Read the model definition and answer for the solid it produces. Units are mm, in the model's axes. A direction names the side the tool comes from. Round coordinates to 2 decimals unless told otherwise and drop trailing zeros. Write each loop counter-clockwise with the first axis right and the second up, starting at its lowest first coordinate (ties: lowest second). Pieces come first, ordered by that corner, then holes. Notation, with made-up numbers: (34, 14.25) - (54, 14.25) arc R25 cw to (54, 35.25) - close; hole circle Ø1 at (-36.75, 25.5). An arc over 180 degrees is marked (long way). One line per item, written item: value. Start each with the question number.
(1) A cutting plane is placed at A-A, the plane x = 9.5. State how many separate pieces and enclosed holes the cut face has, plus the area to 3 significant figures.
(2) Find the intervals of material crossed by L1, parallel to Y at x = 80, z = 93.5; L2, parallel to X at y = 147, z = 83; L3, parallel to Z at x = 20, y = 40.5, in increasing order.
(3) The mould has two halves that part along Y. Classify faces 3 (the face through (76, 85, 33)), 4 (the face through (0, 78, 63)), 5 (the face through (41, 0, 63)): +Y half, -Y half, draft (parallel to the pull), parting line (faces both ways), or undercut.
(4) A cutting plane is placed at D-D, the plane x = 68. Determine the outline of the cut face in (y, z).
(5) A cutting plane is placed at C-C, the plane y = 125.5. Determine the outline of the cut face in (x, z), plus the area to 3 significant figures.
(6) A cutting plane is placed at B-B, the plane z = 8. Determine the outline of the cut face in (x, y), plus the area to 3 significant figures.
(7) For faces 1 (the face through (76, 124, 33)), 2 (the face through (41, 157.8, 63)), determine the directions among +Z, -Z, +X, -X, +Y, -Y from which every point of the face is accessible in a straight line to the end or side of a thin tool.
(8) Flat-ended cylindrical pins translate along their axes: pin 1 Ø11 at (x, y) = (74, 125.5) entering from +Z; pin 2 Ø12 at (x, y) = (43, 129) entering from +Z; pin 3 Ø1.5 at (x, y) = (44, 1) entering from +Z. Find the tip coordinate at first contact, or state that the pin passes through.
from build123d import *

# Parameters (mm, degrees)
SKETCH1_W           = 83.5
SKETCH1_H           = 157.8
SKETCH1_W_2         = 77.5
SKETCH1_H_2         = 35.7
BOSS_EXTRUDE1_DEPTH = 123
SKETCH1_3_W         = 77.5
SKETCH1_3_H         = 35.7
BOSS_EXTRUDE2_DEPTH = 3
SKETCH2_W           = 77.5
SKETCH2_H           = 27
CUT_EXTRUDE1_DEPTH  = 100
SKETCH4_W           = 3
SKETCH4_H           = 10
BOSS_EXTRUDE3_DEPTH = 10
SKETCH5_W           = 3
SKETCH5_H           = 10
BOSS_EXTRUDE4_DEPTH = 10
SKETCH7_W           = 3
SKETCH7_H           = 157.8
BOSS_EXTRUDE5_DEPTH = 5
SKETCH8_W           = 1
SKETCH8_H           = 2.5
CUT_EXTRUDE2_DEPTH  = 154.8
SKETCH9_W           = 7.5
SKETCH9_H           = 7.5
CUT_EXTRUDE3_DEPTH  = 10


with BuildPart() as part:
    # Sketch1 → Boss-Extrude1 (new body)
    with BuildSketch(Plane.XY):
        with Locations((41.75, 78.9)):
            Rectangle(SKETCH1_W, SKETCH1_H)
        with Locations((41.75, 20.85)):
            Rectangle(SKETCH1_W_2, SKETCH1_H_2, mode=Mode.SUBTRACT)
        with Locations((41.75, 59.55)):
            Rectangle(SKETCH1_W_2, SKETCH1_H_2, mode=Mode.SUBTRACT)
        with Locations((41.75, 98.25)):
            Rectangle(SKETCH1_W_2, SKETCH1_H_2, mode=Mode.SUBTRACT)
        with Locations((41.75, 136.95)):
            Rectangle(SKETCH1_W_2, SKETCH1_H_2, mode=Mode.SUBTRACT)
    extrude(amount=BOSS_EXTRUDE1_DEPTH)

    # Sketch1<3> → Boss-Extrude2 (add)
    with BuildSketch(Plane.XY):
        with Locations((41.75, 136.95)):
            Rectangle(SKETCH1_3_W, SKETCH1_3_H)
        with Locations((41.75, 98.25)):
            Rectangle(SKETCH1_3_W, SKETCH1_3_H)
        with Locations((41.75, 59.55)):
            Rectangle(SKETCH1_3_W, SKETCH1_3_H)
        with Locations((41.75, 20.85)):
            Rectangle(SKETCH1_3_W, SKETCH1_3_H)
    extrude(amount=BOSS_EXTRUDE2_DEPTH)

    # Sketch2 → Cut-Extrude1 (cut)
    with BuildSketch(Plane(origin=(0, 119.1, 0), x_dir=(1, 0, 0), z_dir=(0, 1, 0))):
        with Locations((41.75, -16.5)):
            Rectangle(SKETCH2_W, SKETCH2_H)
    extrude(amount=-CUT_EXTRUDE1_DEPTH, mode=Mode.SUBTRACT)

    # Sketch4 → Boss-Extrude3 (add)
    with BuildSketch(Plane(origin=(3, 0, 0), x_dir=(0, 0, -1), z_dir=(1, 0, 0))):
        with Locations((-31.5, 85.4)):
            Rectangle(SKETCH4_W, SKETCH4_H)
        with Locations((-31.5, 124.1)):
            Rectangle(SKETCH4_W, SKETCH4_H)
        with Locations((-31.5, 46.7)):
            Rectangle(SKETCH4_W, SKETCH4_H)
        with Locations((-31.5, 8)):
            Rectangle(SKETCH4_W, SKETCH4_H)
    extrude(amount=BOSS_EXTRUDE3_DEPTH)

    # Sketch5 → Boss-Extrude4 (add)
    with BuildSketch(Plane.ZY.offset(-80.5)):
        with Locations((31.5, 85.4)):
            Rectangle(SKETCH5_W, SKETCH5_H)
        with Locations((31.5, 124.1)):
            Rectangle(SKETCH5_W, SKETCH5_H)
        with Locations((31.5, 46.7)):
            Rectangle(SKETCH5_W, SKETCH5_H)
        with Locations((31.5, 8)):
            Rectangle(SKETCH5_W, SKETCH5_H)
    extrude(amount=BOSS_EXTRUDE4_DEPTH)

    # Sketch7 → Boss-Extrude5 (add)
    with BuildSketch(Plane.XY.offset(123)):
        with Locations((1.5, 78.9)):
            Rectangle(SKETCH7_W, SKETCH7_H)
        with Locations((82, 78.9)):
            Rectangle(SKETCH7_W, SKETCH7_H)
    extrude(amount=BOSS_EXTRUDE5_DEPTH)

    # Sketch8 → Cut-Extrude2 (cut)
    with BuildSketch(Plane(origin=(0, 157.8, 0), x_dir=(1, 0, 0), z_dir=(0, 1, 0))):
        with Locations((2.5, -124.25)):
            Rectangle(SKETCH8_W, SKETCH8_H)
        with Locations((81, -124.25)):
            Rectangle(SKETCH8_W, SKETCH8_H)
    extrude(amount=-CUT_EXTRUDE2_DEPTH, mode=Mode.SUBTRACT)

    # Sketch9 → Cut-Extrude3 (cut)
    with BuildSketch(Plane(origin=(0, 157.8, 0), x_dir=(1, 0, 0), z_dir=(0, 1, 0))):
        with Locations((69.75, -13.75)):
            Rectangle(SKETCH9_W, SKETCH9_H)
    extrude(amount=-CUT_EXTRUDE3_DEPTH, mode=Mode.SUBTRACT)


solid = part.part
Here are the results:
1. separate pieces: 4
1. enclosed holes: 0
1. area: 2,150 mm²
2. L1: 0 to 3, 38.7 to 41.7, 77.4 to 80.4, 116.1 to 119.1, 154.8 to 157.8
2. L2: 0 to 3, 80.5 to 83.5
2. L3: 0 to 3, 30 to 123
3. face 3: undercut
3. face 4: draft
3. face 5: -Y half
4. outline: (0, 0) - (157.8, 0) - (157.8, 10) - (154.8, 10) - (154.8, 3) - (3, 3) - (3, 123) - (0, 123) - close; (38.7, 30) - (41.7, 30) - (41.7, 123) - (38.7, 123) - close; (77.4, 30) - (80.4, 30) - (80.4, 123) - (77.4, 123) - close; (116.1, 30) - (119.1, 30) - (119.1, 123) - (116.1, 123) - close; (154.8, 17.5) - (157.8, 17.5) - (157.8, 123) - (154.8, 123) - close
5. outline: (0, 0) - (83.5, 0) - (83.5, 128) - (80.5, 128) - (80.5, 125.5) - (81.5, 125.5) - (81.5, 123) - (80.5, 123) - (80.5, 33) - (70.5, 33) - (70.5, 30) - (80.5, 30) - (80.5, 3) - (3, 3) - (3, 30) - (13, 30) - (13, 33) - (3, 33) - (3, 123) - (2, 123) - (2, 125.5) - (3, 125.5) - (3, 128) - (0, 128) - close
5. area: 1,060 mm²
6. outline: (0, 0) - (83.5, 0) - (83.5, 157.8) - (0, 157.8) - close; hole (3, 3) - (80.5, 3) - (80.5, 154.8) - (3, 154.8) - close
6. area: 1,410 mm²
7. face 1: +Z
7. face 2: +Z, -Z, +X, -X, +Y
8. pin 1: z = 33
8. pin 2: z = 3
8. pin 3: z = 123
